```python
from build123d import *
from OCP.BRepFilletAPI import BRepFilletAPI_MakeFillet

# Parameters (mm, degrees)
SKETCH1_W            = 290
SKETCH1_H            = 140
MAIN_BODY_DEPTH      = 10
SKETCH2_W            = 164.64
SKETCH2_H            = 99.6
DISPLAY_DEPTH        = 10
SKETCH5_W            = 10
SKETCH5_H            = 10
FEET_DEPTH           = 10
FEET_FILLETS_R1      = 5
FEET_FILLETS_R2      = 1
SKETCH8_R            = 10
ROTARY_ENCODER_DEPTH = 10
SKETCH9_R            = 13.5
CONNECTORS_DEPTH     = 10
SNAP_START           = 285.5
SNAP_HOOK1_DEPTH     = 2
SNAP_START_2         = -26.59133039
SNAP_HOOK1_2_DEPTH   = 7.70946078
SNAP_START_3         = 287.5
SNAP_HOOK1_3_DEPTH   = 3.5
SNAP_HOOK2_DEPTH     = 2
SNAP_START_4         = -121.11813039
SNAP_HOOK2_2_DEPTH   = 7.70946078
SNAP_HOOK2_3_DEPTH   = 3.5
SNAP_START_5         = 2.5
SNAP_HOOK3_DEPTH     = 2
SNAP_HOOK3_2_DEPTH   = 7.70946078
SNAP_START_6         = -1
SNAP_HOOK3_3_DEPTH   = 3.5
SNAP_HOOK4_DEPTH     = 2
SNAP_HOOK4_2_DEPTH   = 7.70946078
SNAP_HOOK4_3_DEPTH   = 3.5
SIDE_FILLETS_R       = 5.7366
SKETCH11_R           = 1.5
DISPLAY_HOLES_DEPTH  = 7


with BuildPart() as part:
    # Sketch1 → Main Body (new body)
    with BuildSketch(Plane.XY):
        with Locations((145, -70)):
            Rectangle(SKETCH1_W, SKETCH1_H)
    extrude(amount=MAIN_BODY_DEPTH)

    # Sketch2 → Display (cut)
    with BuildSketch(Plane(origin=(0, 0, 0), x_dir=(-1, 0, 0), z_dir=(0, 0, -1))):
        with Locations((-107.32, -69.3)):
            Rectangle(SKETCH2_W, SKETCH2_H)
    extrude(amount=-DISPLAY_DEPTH, mode=Mode.SUBTRACT)

    # Sketch5 → Feet (add)
    with BuildSketch(Plane.XZ.offset(140)):
        with Locations((20, 5)):
            Rectangle(SKETCH5_W, SKETCH5_H)
        with Locations((270, 5)):
            Rectangle(SKETCH5_W, SKETCH5_H)
    extrude(amount=FEET_DEPTH)

    # Feet Fillets: one fillet with a radius per group of edges: ONE call of the kernel's fillet builder (fillet() takes one radius for all edges)
    feet_fillets_edges_1 = [part.edges().sort_by_distance(p)[0] for p in [
        (15, -140, 5),
        (25, -140, 5),
        (275, -140, 5),
        (265, -140, 5),
    ]]
    feet_fillets_edges_2 = [part.edges().sort_by_distance(p)[0] for p in [
        (265, -150, 5),
        (275, -150, 5),
        (25, -150, 5),
        (15, -150, 5),
    ]]
    feet_fillets = BRepFilletAPI_MakeFillet(part.part.solid().wrapped)
    for e in feet_fillets_edges_1:
        feet_fillets.Add(FEET_FILLETS_R1, e.wrapped)
    for e in feet_fillets_edges_2:
        feet_fillets.Add(FEET_FILLETS_R2, e.wrapped)
    add(Compound.cast(feet_fillets.Shape()), mode=Mode.REPLACE)

    # Sketch8 → Rotary Encoder (cut)
    with BuildSketch(Plane.XY.offset(10)):
        with Locations((239.82, -29.550599566)):
            Circle(SKETCH8_R)
    extrude(amount=-ROTARY_ENCODER_DEPTH, mode=Mode.SUBTRACT)

    # Sketch9 → Connectors (cut)
    with BuildSketch(Plane.XY.offset(10)):
        with Locations((214.961120299, -93.741529743)):
            Circle(SKETCH9_R)
        with Locations((264.678879701, -93.741529743)):
            Circle(SKETCH9_R)
    extrude(amount=-CONNECTORS_DEPTH, mode=Mode.SUBTRACT)

    # Snap Hook1: read off the stored shape, not the designer's step
    # Snap Hook1 outline → Snap Hook1 (add)
    with BuildSketch(Plane.YZ.offset(SNAP_START)):
        Polygon((-26.4866, -21), (-18.9866, -21), (-18.620043637, 0), (-26.853156363, 0), align=None)
    extrude(amount=SNAP_HOOK1_DEPTH)

    # Snap Hook1 2 outline → Snap Hook1 2 (add)
    with BuildSketch(Plane(origin=(0, 0, 0), x_dir=(1, 0, 0), z_dir=(0, 1, 0)).offset(SNAP_START_2)):
        Polygon((287.5, 15), (290.5, 15), (287.5, 21), align=None)
    extrude(amount=SNAP_HOOK1_2_DEPTH)

    # Snap Hook1 3 outline → Snap Hook1 3 (cut)
    with BuildSketch(Plane.YZ.offset(SNAP_START_3)):
        Polygon((-18.881869611, -15), (-18.9866, -21), (-19.004055065, -22), (-18.88186961, -22), align=None)
        Polygon((-26.59133039, -22), (-26.469144935, -22), (-26.4866, -21), (-26.591330389, -15), align=None)
    extrude(amount=SNAP_HOOK1_3_DEPTH, mode=Mode.SUBTRACT)

    # Snap Hook2: read off the stored shape, not the designer's step
    # Snap Hook2 outline → Snap Hook2 (add)
    with BuildSketch(Plane.YZ.offset(SNAP_START)):
        Polygon((-121.0134, -21), (-113.5134, -21), (-113.146843637, 0), (-121.379956363, 0), align=None)
    extrude(amount=SNAP_HOOK2_DEPTH)

    # Snap Hook2 2 outline → Snap Hook2 2 (add)
    with BuildSketch(Plane(origin=(0, 0, 0), x_dir=(1, 0, 0), z_dir=(0, 1, 0)).offset(SNAP_START_4)):
        Polygon((287.5, 15), (290.5, 15), (287.5, 21), align=None)
    extrude(amount=SNAP_HOOK2_2_DEPTH)

    # Snap Hook2 3 outline → Snap Hook2 3 (cut)
    with BuildSketch(Plane.YZ.offset(SNAP_START_3)):
        Polygon((-113.408669611, -15), (-113.5134, -21), (-113.530855065, -22), (-113.40866961, -22), align=None)
        Polygon((-121.11813039, -22), (-120.995944935, -22), (-121.0134, -21), (-121.118130389, -15), align=None)
    extrude(amount=SNAP_HOOK2_3_DEPTH, mode=Mode.SUBTRACT)

    # Snap Hook3: read off the stored shape, not the designer's step
    # Snap Hook3 outline → Snap Hook3 (add)
    with BuildSketch(Plane.YZ.offset(SNAP_START_5)):
        Polygon((-26.4866, -21), (-18.9866, -21), (-18.620043637, 0), (-26.853156363, 0), align=None)
    extrude(amount=SNAP_HOOK3_DEPTH)

    # Snap Hook3 2 outline → Snap Hook3 2 (add)
    with BuildSketch(Plane(origin=(0, 0, 0), x_dir=(1, 0, 0), z_dir=(0, 1, 0)).offset(SNAP_START_2)):
        Polygon((2.5, 21), (-0.5, 15), (2.5, 15), align=None)
    extrude(amount=SNAP_HOOK3_2_DEPTH)

    # Snap Hook3 3 outline → Snap Hook3 3 (cut)
    with BuildSketch(Plane.YZ.offset(SNAP_START_6)):
        Polygon((-18.881869611, -15), (-18.9866, -21), (-19.004055065, -22), (-18.88186961, -22), align=None)
        Polygon((-26.59133039, -22), (-26.469144935, -22), (-26.4866, -21), (-26.591330389, -15), align=None)
    extrude(amount=SNAP_HOOK3_3_DEPTH, mode=Mode.SUBTRACT)

    # Snap Hook4: read off the stored shape, not the designer's step
    # Snap Hook4 outline → Snap Hook4 (add)
    with BuildSketch(Plane.YZ.offset(SNAP_START_5)):
        Polygon((-121.0134, -21), (-113.5134, -21), (-113.146843637, 0), (-121.379956363, 0), align=None)
    extrude(amount=SNAP_HOOK4_DEPTH)

    # Snap Hook4 2 outline → Snap Hook4 2 (add)
    with BuildSketch(Plane(origin=(0, 0, 0), x_dir=(1, 0, 0), z_dir=(0, 1, 0)).offset(SNAP_START_4)):
        Polygon((2.5, 21), (-0.5, 15), (2.5, 15), align=None)
    extrude(amount=SNAP_HOOK4_2_DEPTH)

    # Snap Hook4 3 outline → Snap Hook4 3 (cut)
    with BuildSketch(Plane.YZ.offset(SNAP_START_6)):
        Polygon((-113.408669611, -15), (-113.5134, -21), (-113.530855065, -22), (-113.40866961, -22), align=None)
        Polygon((-121.11813039, -22), (-120.995944935, -22), (-121.0134, -21), (-121.118130389, -15), align=None)
    extrude(amount=SNAP_HOOK4_3_DEPTH, mode=Mode.SUBTRACT)

    # Side Fillets
    side_fillets_edges = [part.edges().sort_by_distance(p)[0] for p in [
        (0, 0, 5),
        (290, 0, 5),
        (290, -140, 5),
        (0, -140, 5),
    ]]
    fillet(side_fillets_edges, radius=SIDE_FILLETS_R)

    # Sketch11 → Display Holes (cut)
    with BuildSketch(Plane(origin=(0, 0, 0), x_dir=(-1, 0, 0), z_dir=(0, 0, -1))):
        with Locations((-185.77, -11.82)):
            Circle(SKETCH11_R)
        with Locations((-28.87, -11.82)):
            Circle(SKETCH11_R)
        with Locations((-185.77, -126.78)):
            Circle(SKETCH11_R)
        with Locations((-28.87, -126.78)):
            Circle(SKETCH11_R)
    extrude(amount=-DISPLAY_HOLES_DEPTH, mode=Mode.SUBTRACT)


solid = part.part
```
Geometry check sheet. Reference: the model listing, model coordinates, mm. A direction names the side the tool comes from. Coordinates: 2 decimals unless noted, no trailing zeros. Loops run counter-clockwise (first coordinate to the right, second up) from the corner with the lowest first, then second, coordinate; pieces in that order, holes last. Notation, with made-up numbers: (-3.5, 40) - (4.5, 40) arc R9 ccw to (4.5, 57) - close; hole circle Ø4 at (-20.75, 16). An arc over 180 degrees is marked (long way). One line per item, written item: value. Start each with the question number.
(1) Cross-section at A-A on x = 138. Enter the section's corners in (y, z).
(2) Mould release check, pull along X, two halves, no side actions. Record for faces 1 (the flat face through (287.5, -23, -7)), 2 (the flat face through (108, -19.5, 5)), 3 (the flat face through (20, -150, 5)): released by +X, released by -X, zero draft, split by the parting line, or undercut.
(3) Tool access check on faces 4 (the flat face through (25, -70, 5)), 5 (the flat face through (285.5, -117, -10)), 6 (the flat face through (289, -23, -18)). Record the directions out of +Z, -Z, +X, -X, +Y, -Y that give a thin tool (end or side, any length) a straight path to the whole face; none if there is none.
(4) Cross-section at B-B on y = -70. Enter the section's corners in (x, z).
(5) Cross-section at C-C on z = -9. Enter the section's corners in (x, y).
(6) Material ranges on line 1 (X direction, y = -11, z = 2); line 2 (X direction, y = -126.78, z = 5.25); line 3 (Y direction, x = 47, z = 0.5), recorded low to high. Write a range as [from, to].
(7) Depth check by flat-ended pin: P1, Ø4.5, axis at x = 282, z = 4, coming from the -Y side; P2, Ø2, axis at y = -147, z = 6, coming from the -X side; P3, Ø3, axis at y = -84, z = 3.5, coming from the +X side. Enter the tip coordinate at first touch or a pass-through.
Results below:
1. outline: (-140, 0) - (-119.1, 0) - (-119.1, 10) - (-140, 10) - close; (-19.5, 0) - (0, 0) - (0, 10) - (-19.5, 10) - close
2. face 1: released by +X
2. face 2: undercut
2. face 3: zero draft
3. face 4: +Z, -Z
3. face 5: -Z, +Y, -Y
3. face 6: -Z, +X, +Y, -Y
4. outline: (0, 0) - (25, 0) - (25, 10) - (0, 10) - close; (189.64, 0) - (290, 0) - (290, 10) - (189.64, 10) - close
5. outline: (2.5, -121.22) - (4.5, -121.22) - (4.5, -113.3) - (2.5, -113.3) - close; (2.5, -26.7) - (4.5, -26.7) - (4.5, -18.78) - (2.5, -18.78) - close; (285.5, -121.22) - (287.5, -121.22) - (287.5, -113.3) - (285.5, -113.3) - close; (285.5, -26.7) - (287.5, -26.7) - (287.5, -18.78) - (285.5, -18.78) - close
6. line 1: x = [0, 27.61], [30.13, 184.51], [187.03, 290]
6. line 2: x = [0, 27.37], [30.37, 184.27], [187.27, 290]
6. line 3: y = [-140, -119.1], [-19.5, 0]
7. P1: stops at y = -140.01
7. P2: stops at x = 15
7. P3: stops at x = 290
